Source: CAD feature listing. Evaluate the final solid. Frame: model axes, mm. A direction names the side the tool comes from. Round coordinates to 2 decimals unless told otherwise and drop trailing zeros. Loops run counter-clockwise (first coordinate to the right, second up) from the corner with the lowest first, then second, coordinate; pieces in that order, holes last. Notation, with made-up numbers: (-35.75, -22.75) -> (-14.75, -22.75) arc R20 ccw to (-14.75, -16.75) -> close; hole circle Ø11 at (-23, -13.5). An arc over 180 degrees is marked (long way). Put each result on its own line as item: value. Start each with the question number.
1. Contact query for flat-ended pins moving along their axis: pin 1 (1 mm diameter, centred on y = 48, z = 5, fed in from +X); pin 2 (4 mm diameter, centred on x = 17.5, z = 14.5, fed in from -Y); pin 3 (1 mm diameter, centred on y = 13.5, z = 11, fed in from -X). Output: stop coordinate, or through.
2. Draft query along Z for faces 1 (the flat face through (2, 0, 9)), 2 (the cylindrical face through (2.535, 31.715, 9.225)). Return one class per face: pulls with the +Z half, pulls with the -Z half, needs draft (parallel to the pull), parting line crosses it, or undercut.
3. Cut plane A-A (z = 9). Return the cut outline in (x, y), then the cut area to 3 significant figures.
4. Cut plane D-D (x = 30). Return the cut outline in (y, z), then the cut area to 3 significant figures.
5. Material intervals for L1, parallel to Z at x = 1, y = 4; L2, parallel to X at y = 45.5, z = 3.25; L3, parallel to Y at x = 30, z = 9.25, sorted ascending.
6. Cut plane B-B (y = 4). Return the cut outline in (x, z).
7. Set-up query: faces 3 (the flat face through (30, 50, 9)), 4 (the flat face through (0, 28, 9)). Return all of +Z, -Z, +X, -X, +Y, -Y with unobstructed straight access to the full face (end or side cutting, diameter ignored); none if empty.
8. Cut plane C-C (z = 4.5). Return the cut outline in (x, y), then the cut area to 3 significant figures.
```python
from build123d import *

# Parameters (mm, degrees)
PAD_DEPTH    = 18
SKETCH001_R  = 0.75
POCKET_DEPTH = 5.001


with BuildPart() as part:
    # Sketch → Pad (new body)
    with BuildSketch(Plane.XY):
        Polygon((5, 0), (5, 50), (55, 50), (55, 55), (0, 55), (0, 0), align=None)
    extrude(amount=PAD_DEPTH)

    # Sketch001 (on Face2 of Pad) → Pocket (cut, through all)
    with BuildSketch(Plane.YZ.offset(5)):
        with Locations((4, 9)):
            Circle(SKETCH001_R)
        with Locations((31, 9)):
            Circle(SKETCH001_R)
    extrude(amount=-POCKET_DEPTH, mode=Mode.SUBTRACT)


solid = part.part
```
Solution:
1. pin 1: stops at x = 5
1. pin 2: stops at y = 50
1. pin 3: stops at x = 0
2. face 1: needs draft
2. face 2: undercut
3. outline: (0, 0) -> (5, 0) -> (5, 3.25) -> (0, 3.25) -> close; (0, 4.75) -> (5, 4.75) -> (5, 30.25) -> (0, 30.25) -> close; (0, 31.75) -> (5, 31.75) -> (5, 50) -> (55, 50) -> (55, 55) -> (0, 55) -> close
3. area: 510 mm^2
4. outline: (50, 0) -> (55, 0) -> (55, 18) -> (50, 18) -> close
4. area: 90.0 mm^2
5. L1: z = 0 to 8.25, 9.75 to 18
5. L2: x = 0 to 5
5. L3: y = 50 to 55
6. outline: (0, 0) -> (5, 0) -> (5, 8.25) -> (0, 8.25) -> close; (0, 9.75) -> (5, 9.75) -> (5, 18) -> (0, 18) -> close
7. face 3: +Z, -Z, +X, -Y
7. face 4: +Z, -Z, -X, +Y, -Y
8. outline: (0, 0) -> (5, 0) -> (5, 50) -> (55, 50) -> (55, 55) -> (0, 55) -> close
8. area: 525 mm^2
